```python
from build123d import *

# Parameters (mm, degrees)
SKETCH2_W           = 254
SKETCH2_H           = 254
BOSS_EXTRUDE1_DEPTH = 127
SKETCH3_R           = 44.45
CUT_EXTRUDE1_DEPTH  = 82.55
FILLET1_R           = 12.7


with BuildPart() as part:
    # Sketch2 → Boss-Extrude1 (new body, symmetric)
    with BuildSketch(Plane.XY):
        Rectangle(SKETCH2_W, SKETCH2_H)
    extrude(amount=BOSS_EXTRUDE1_DEPTH, both=True)

    # Sketch3 → Cut-Extrude1 (cut)
    with BuildSketch(Plane(origin=(0, 127, 0), x_dir=(1, 0, 0), z_dir=(0, 1, 0))):
        Circle(SKETCH3_R)
    extrude(amount=-CUT_EXTRUDE1_DEPTH, mode=Mode.SUBTRACT)

    # Fillet1
    fillet1_edges = [part.edges().sort_by_distance(p)[0] for p in [
        (0, 127, 127),
        (0, 127, -127),
        (-127, 127, 0),
        (127, 127, 0),
    ]]
    fillet(fillet1_edges, radius=FILLET1_R)


solid = part.part
```
Check sheet for the modelled part. Datum: model origin and axes. Units: mm. Give positions to 0.01 mm unless a question says otherwise; leave off trailing zeros. Order: outer loops, then holes, each group sorted by start corner. A loop starts at its lowest first (then second) coordinate and runs counter-clockwise, first axis right, second up. Notation, with made-up numbers: (-11.5, 72) -> (21.5, 72) arc R23 ccw to (21.5, 87) -> close; hole circle Ø2 at (-2, 47). An arc over 180 degrees is marked (long way). Return JSON: item names as keys, results as strings.
1. Cross-section at A-A, the plane x = 0. Record the cut outline in (y, z).
From the geometry:
{"outline": "(-127, -127) -> (114.3, -127) arc R12.7 ccw to (127, -114.3) -> (127, -44.45) -> (44.45, -44.45) -> (44.45, 44.45) -> (127, 44.45) -> (127, 114.3) arc R12.7 ccw to (114.3, 127) -> (-127, 127) -> close"}
2. Material ranges on probe 1 along Z at (x, y) = (0, 91); probe 2 along Y at (x, z) = (-30.5, -31), recorded low to high. Write a range as [from, to].
From the geometry:
{"probe 1": "[-127, -44.45], [44.45, 127]", "probe 2": "[-127, 44.45]"}
3. Mould release check, pull along Z, two halves, no side actions. Record for faces 1 (the flat face through (-1, 44.45, -1)), 2 (the cylindrical face through (42.397, 86.303, -13.352)), 3 (the flat face through (-2, -5, -127)), 4 (the flat face through (127, -8, 2)): +Z half, -Z half, draft (parallel to the pull), parting line (faces both ways), or undercut.
From the geometry:
{"face 1": "undercut", "face 2": "undercut", "face 3": "-Z half", "face 4": "draft"}
4. Cross-section at B-B, the plane z = 0. Record the cut outline in (x, y).
From the geometry:
{"outline": "(-127, -127) -> (127, -127) -> (127, 114.3) arc R12.7 ccw to (114.3, 127) -> (44.45, 127) -> (44.45, 44.45) -> (-44.45, 44.45) -> (-44.45, 127) -> (-114.3, 127) arc R12.7 ccw to (-127, 114.3) -> close"}
